from build123d import *

# Parameters (mm, degrees)
F0_R      = 31.75
F1_DEPTH  = 93.853
F2_R      = 21.2471
F3_DEPTH  = 1.5748
F5_DEPTH  = 23.7998
F7_DEPTH  = 23.7998
F8_R      = 1.7018
F9_DEPTH  = 12.7
F10_DEPTH = 12.7
F11_R     = 0.635
F12_R     = 0.635
F13_R     = 0.635
F14_R     = 6.35
F15_DEPTH = 25.4
F16_R     = 6.35
F17_DEPTH = 25.4


with BuildPart() as f1:
    # F0 (on Top) → F1 (new body)
    with BuildSketch(Plane.XY):
        Circle(F0_R)
    extrude(amount=F1_DEPTH)

    # F2 (on face) → F3 (join)
    with BuildSketch(Plane.XY.offset(93.853)):
        Circle(F2_R)
    extrude(amount=F3_DEPTH)

    # F4 (on face) → F5 (cut)
    with BuildSketch(Plane.XY.offset(93.853)):
        with BuildLine():
            Line((-9.6392581686, 30.2514), (9.6392581686, 30.2514))
            ThreePointArc((9.6392581686, 30.2514), (0, 31.75), (-9.6392581686, 30.2514))
        make_face()
    extrude(amount=-F5_DEPTH, mode=Mode.SUBTRACT)

    # F6 (on face) → F7 (cut, through all)
    with BuildSketch(Plane.XY.offset(93.853)):
        with BuildLine():
            Line((-31.0418451257, 6.6683094701), (-21.4615892087, 23.397920605))
            ThreePointArc((-21.4615892087, 23.397920605), (-27.5521800663, 15.7778285449), (-31.0418451257, 6.6683094701))
        make_face()
    extrude(amount=-F7_DEPTH, mode=Mode.SUBTRACT)

    # F8 (on face) → F9 (cut)
    with BuildSketch(Plane.XY.offset(93.853)):
        with Locations((-10.738599221, -24.3847738544)):
            Circle(F8_R)
    extrude(amount=-F9_DEPTH, mode=Mode.SUBTRACT)

    # F8 (on face) → F10 (cut)
    with BuildSketch(Plane.XY.offset(93.853)):
        with Locations((26.4903553103, -2.8628280933)):
            Circle(F8_R)
    extrude(amount=-F10_DEPTH, mode=Mode.SUBTRACT)

    # F11
    f11_edges = [f1.edges().sort_by_distance(p)[0] for p in [
        (-3.352903, -31.572465, 93.853),
    ]]
    fillet(f11_edges, radius=F11_R)

    # F12
    f12_edges = [f1.edges().sort_by_distance(p)[0] for p in [
        (-15.923512, 27.468241, 93.853),
    ]]
    fillet(f12_edges, radius=F12_R)

    # F13
    f13_edges = [f1.edges().sort_by_distance(p)[0] for p in [
        (-31.75, 0, 0),
    ]]
    fillet(f13_edges, radius=F13_R)

    # F14 (on face) → F15 (cut)
    with BuildSketch(Plane(origin=(0, 30.2514, 0), x_dir=(-1, 0, 0), z_dir=(0, 1, 0))):
        with Locations((0, 81.9531)):
            Circle(F14_R)
    extrude(amount=-F15_DEPTH, mode=Mode.SUBTRACT)

    # F16 (on face) → F17 (cut)
    with BuildSketch(Plane(origin=(-26.2517171672, 15.0331150376, 0), x_dir=(-0.4969394817, -0.8677851989, 0), z_dir=(-0.8677851989, 0.4969394817, 0))):
        with Locations((-0.1142581686, 81.9531)):
            Circle(F16_R)
    extrude(amount=-F17_DEPTH, mode=Mode.SUBTRACT)

    # F20 (on Front) → F21 (revolve, cut)
    with BuildSketch(Plane.XZ):
        Polygon((31.75, 69.6722), (31.75, 70.4342), (31.369, 70.0532), align=None)
    revolve(axis=Axis((0, 0, 0), (0, 0, -1)), mode=Mode.SUBTRACT)


solid = f1.part
Design review of the part built by this model. Coordinates are the model's own, in mm. A direction names the side the tool comes from. Give positions to 0.01 mm unless a question says otherwise; leave off trailing zeros. Loops run counter-clockwise (first coordinate to the right, second up) from the corner with the lowest first, then second, coordinate; pieces in that order, holes last. Notation, with made-up numbers: (7, -32.5) -> (53, -32.5) arc R14 ccw to (53, -14.5) -> close; hole circle Ø7 at (41, 39.5). An arc over 180 degrees is marked (long way). One line per question, with ' | ' between items. Start each with the question number.
(1) We need section B-B (z = 58). State the section outline as (x, y) points.
(2) Draft analysis for pull direction X (two halves, no side actions). For faces 1 (the face through (-27, 15, 70.053)), 2 (the face through (-18.24, 3.82, 79.52)), 3 (the face through (-6.883, -30.995, 34.67)), state which applies: +X half, -X half, draft (parallel to the pull), parting line (faces both ways), or undercut.
(3) For line 1 (Z direction, x = 0, y = 25); line 2 (Z direction, x = 29, y = 2.5); line 3 (Y direction, x = 1, z = 22), list the stretches that pass through material, from the lowest coordinate up.
(4) For faces 4 (the face through (-29.51, 9.34, 82.12)), 5 (the face through (-9.953, -25.895, 87.592)), 6 (the face through (-7, 30.251, 82)), 7 (the face through (1, 4.851, 82)), list the 3-axis set-ups (+Z, -Z, +X, -X, +Y, -Y) from which the entire face can be reached by the end or side of a thin tool; tool diameter is ignored.
(5) We need section A-A (x = 0). State the section outline as (y, z) points (3 decimals), and give its area (3 significant figures).
(6) Insertion check: P1, Ø11.5, axis at x = 0, z = 81.95, coming from the +Y side; P2, Ø1, axis at x = 26, y = -3, coming from the +Z side; P3, Ø2, axis at x = -9.5, z = 79, coming from the +Y side. Each pin has a flat end and moves straight along its axis. Give the tip position at first contact, or say it passes through.
The answers:
1) outline: circle Ø63.5 at (0, 0)
2) face 1: draft | face 2: undercut | face 3: parting line
3) line 1: z = 0 to 75.6, 88.3 to 93.85 | line 2: z = 0 to 93.85 | line 3: y = -31.73 to 31.73
4) face 4: +Z, -X, +Y | face 5: +Z | face 6: +Z, +X, -X, +Y | face 7: +Y
5) outline: (-31.75, 0.635) arc R0.635 ccw to (-31.115, 0) -> (31.115, 0) arc R0.635 ccw to (31.75, 0.635) -> (31.75, 69.672) -> (31.369, 70.053) -> (30.251, 70.053) -> (30.251, 75.603) -> (4.851, 75.603) -> (4.851, 88.303) -> (30.251, 88.303) -> (30.251, 93.853) -> (21.247, 93.853) -> (21.247, 95.428) -> (-21.247, 95.428) -> (-21.247, 93.853) -> (-31.115, 93.853) arc R0.635 ccw to (-31.75, 93.218) -> (-31.75, 70.434) -> (-31.369, 70.053) -> (-31.75, 69.672) -> close | area: 5,670 mm^2
6) P1: stops at y = 4.85 | P2: stops at z = 81.15 | P3: stops at y = 30.25
